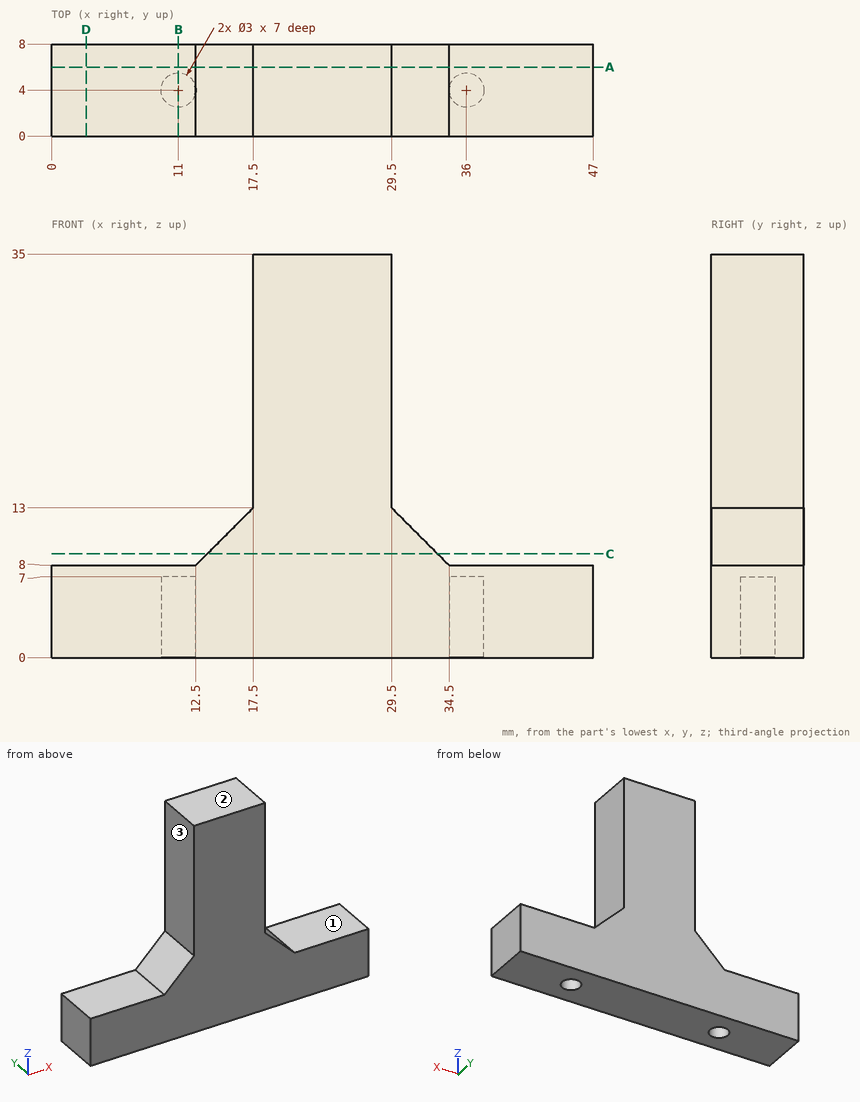
Print and shaded views of the part. All mm, measured from the part's lowest x, y and z. A direction names the side the tool comes from. Coordinates: 2 decimals unless noted, no trailing zeros. Loops run counter-clockwise (first coordinate to the right, second up) from the corner with the lowest first, then second, coordinate; pieces in that order, holes last. Notation, with made-up numbers: (-26, -13) - (2, -13) arc R23 ccw to (2, -1) - close; hole circle Ø3 at (-23, -29.75). An arc over 180 degrees is marked (long way). Write item = value, one per line. Start each with the question number.
Item 1: 3-axis set-ups, long thin cutter, end or side, ignore diameter. For the marked faces 1, 2 and 3: which of +Z, -Z, +X, -X, +Y, -Y reach the whole face in a straight line?
Item 2: Flat gauge pins, fed straight in: pin 1 Ø4 at (y, z) = (6, 21.5) entering from +X; pin 2 Ø4 at (y, z) = (5, 18.5) entering from -X; pin 3 Ø4 at (x, y) = (6, 4.5) entering from +Z. Where does each tip first touch, or does it go through?
Item 3: Cut at C-C, the plane z = 9. Give the cut face in (x, y).
Item 4: Cut at B-B, the plane x = 11. Give the cut face in (y, z).
Item 5: Wall check: L1, parallel to X at y = 4, z = 4.5; L2, parallel to X at y = 3, z = 5; L3, parallel to Y at x = 36, z = 3.5. Give the ranges that are in metal, low to high. Write a range as from..to.
Item 6: Cut at D-D, the plane x = 3. Give the cut face in (y, z), and give its area (3 significant figures).
Item 7: Cut at A-A, the plane y = 6. Give the cut face in (x, z).
The answers:
q1.face_1 = +Z, +X, +Y, -Y
q1.face_2 = +Z, +X, -X, +Y, -Y
q1.face_3 = +Z, -X, +Y, -Y
q2.pin_1 = 29.5
q2.pin_2 = 17.5
q2.pin_3 = 8
q3.outline = (13.5, 0) - (33.5, 0) - (33.5, 8) - (13.5, 8) - close
q4.outline = (0, 0) - (2.5, 0) - (2.5, 7) - (5.5, 7) - (5.5, 0) - (8, 0) - (8, 8) - (0, 8) - close
q5.L1 = 0..9.5, 12.5..34.5, 37.5..47
q5.L2 = 0..9.88, 12.12..34.88, 37.12..47
q5.L3 = 0..2.5, 5.5..8
q6.outline = (0, 0) - (8, 0) - (8, 8) - (0, 8) - close
q6.area = 64.0 mm2
q7.outline = (0, 0) - (47, 0) - (47, 8) - (34.5, 8) - (29.5, 13) - (29.5, 35) - (17.5, 35) - (17.5, 13) - (12.5, 8) - (0, 8) - close
